Check sheet for the modelled part. Datum: model origin and axes. Units: mm. A direction names the side the tool comes from. Round coordinates to 2 decimals unless told otherwise and drop trailing zeros. Order: outer loops, then holes, each group sorted by start corner. A loop starts at its lowest first (then second) coordinate and runs counter-clockwise, first axis right, second up. Notation, with made-up numbers: (1, -15.75) -> (9, -15.75) arc R30 ccw to (9, 8.25) -> close; hole circle Ø6 at (47.25, 79). An arc over 180 degrees is marked (long way). Answer in a Markdown table with one row per item. Add a question column.
1. Sectioned sample at C-C, the plane y = 20.5. Record the boundary of the cut face in (x, z).
2. Draft check along Y on faces 1 (the flat face through (-1, 2, -41.5)), 2 (the flat face through (-0.97, 32.68, 42.34)), 3 (the flat face through (-1, 17, 36.5)), 4 (the flat face through (-1, 0, -1)). Enter one of: +Y half, -Y half, draft (parallel to the pull), parting line (faces both ways), or undercut.
3. Access from +Z, -Z, +X, -X, +Y, -Y to the whole of each face (thin tool, end or side, straight path). Record for faces 5 (the flat face through (-0.97, 20.21, 0.58)), 6 (the flat face through (-1, 15, 41.5)), 7 (the flat face through (-0.896, 16.278, 4.412)).
4. Depth check by flat-ended pin: P1, Ø12, axis at y = 27.5, z = -4, coming from the +X side; P2, Ø5, axis at x = 53.5, z = -3, coming from the +Y side; P3, Ø15, axis at x = 32.5, y = 20, coming from the +Z side; P4, Ø4, axis at x = 44.5, z = -29, coming from the +Y side. Enter the tip coordinate at first touch or a pass-through.
5. Sectioned sample at B-B, the plane z = 17. Record the boundary of the cut face in (x, y).
6. Sectioned sample at A-A, the plane x = 14.5. Record the boundary of the cut face in (y, z), then the cut area to 3 significant figures.
7. Material ranges on L1, parallel to X at y = 13, z = 12.5; L2, parallel to Y at x = 54.5, z = -8.5; L3, parallel to Y at x = -6, z = 8.5, recorded low to high. Write a range as from..to.
```python
from build123d import *

# Parameters (mm, degrees)
SKETCH1_W           = 138
SKETCH1_H           = 83
BOSS_EXTRUDE1_DEPTH = 5
BOSS_EXTRUDE2_DEPTH = 5
BOSS_EXTRUDE3_DEPTH = 5
SKETCH5_W           = 128
SKETCH5_H           = 25
BOSS_EXTRUDE4_DEPTH = 5
SKETCH7_W           = 138
SKETCH7_H           = 88.255311455
BOSS_EXTRUDE7_DEPTH = 5


with BuildPart() as part:
    # Sketch1 → Boss-Extrude1 (new body)
    with BuildSketch(Plane(origin=(0, 0, 0), x_dir=(1, 0, 0), z_dir=(0, 1, 0))):
        Rectangle(SKETCH1_W, SKETCH1_H)
    extrude(amount=BOSS_EXTRUDE1_DEPTH)

    # Sketch4 → Boss-Extrude3 (add)
    with BuildSketch(Plane.ZY.offset(69)):
        Polygon((41.5, 5), (41.5, 35), (-41.5, 5), align=None)
    extrude(amount=-BOSS_EXTRUDE3_DEPTH)



with BuildPart() as body_2:
    # Sketch2 → Boss-Extrude2 (new body)
    with BuildSketch(Plane(origin=(69, 0, 0), x_dir=(0, 0, -1), z_dir=(1, 0, 0))):
        Polygon((-41.5, 5), (-41.5, 35), (41.5, 5), align=None)
    extrude(amount=-BOSS_EXTRUDE2_DEPTH)


with BuildPart() as part_1:
    add(part.part)

    add(body_2.part)  # Boss-Extrude4 merges body 2
    # Sketch5 → Boss-Extrude4 (add)
    with BuildSketch(Plane.XY.offset(41.5)):
        with Locations((0, 17.5)):
            Rectangle(SKETCH5_W, SKETCH5_H)
    extrude(amount=-BOSS_EXTRUDE4_DEPTH)

    # Sketch7 → Boss-Extrude7 (add)
    with BuildSketch(Plane(origin=(0, 17.689048658, -6.393632045), x_dir=(1, 0, 0), z_dir=(0, 0.9404533124606549, -0.33992288402192333))):
        with Locations((0, -6.798457681)):
            Rectangle(SKETCH7_W, SKETCH7_H)
    extrude(amount=-BOSS_EXTRUDE7_DEPTH)


solid = part_1.part
```
Answer key:
| question | item | result |
|---|---|---|
| 1 | outline | (-69, 1.38) -> (69, 1.38) -> (69, 41.5) -> (-69, 41.5) -> close; hole (-64, 16.09) -> (64, 16.09) -> (64, 36.5) -> (-64, 36.5) -> close |
| 2 | face 1 | draft |
| 2 | face 2 | +Y half |
| 2 | face 3 | undercut |
| 2 | face 4 | -Y half |
| 3 | face 5 | -Z, +X, -X, +Y |
| 3 | face 6 | +Z, +X, -X, -Y |
| 3 | face 7 | none |
| 4 | P1 | passes through |
| 4 | P2 | stops at y = 19.82 |
| 4 | P3 | stops at z = 41.5 |
| 4 | P4 | stops at y = 10.24 |
| 5 | outline | (-69, 0) -> (69, 0) -> (69, 26.14) -> (-69, 26.14) -> close; hole (-64, 5) -> (64, 5) -> (64, 20.83) -> (-64, 20.83) -> close |
| 6 | outline | (0, -41.5) -> (5, -41.5) -> (35, 41.5) -> (30.3, 43.2) -> (29.68, 41.5) -> (0, 41.5) -> close; hole (5, -26.79) -> (27.88, 36.5) -> (5, 36.5) -> close |
| 6 | area | 941 mm² |
| 7 | L1 | x = -69..-64, 64..69 |
| 7 | L2 | y = 0..5, 11.61..16.93 |
| 7 | L3 | y = 0..5, 17.76..23.07 |
